Geometry: final body of the model. Coordinates: model frame, mm. A direction names the side the tool comes from. Give positions to 0.01 mm unless a question says otherwise; leave off trailing zeros. Order: outer loops, then holes, each group sorted by start corner. A loop starts at its lowest first (then second) coordinate and runs counter-clockwise, first axis right, second up. Notation, with made-up numbers: (-2.5, 0.5) -> (3.5, 0.5) arc R12 ccw to (3.5, 19.5) -> close; hole circle Ø1 at (-11, -12). An arc over 180 degrees is marked (long way). One line per item, written item: value. Start each with the question number.
```python
from build123d import *

# Parameters (mm, degrees)
BOSS_EXTRU_1_DEPTH      = 6
ESQUISSE3_R             = 0.625
ENL_V_MAT_EXTRU_4_DEPTH = 6
ESQUISSE4_R             = 0.625
ENL_V_MAT_EXTRU_5_DEPTH = 6


with BuildPart() as part:
    # Esquisse1 → Boss.-Extru.1 (new body)
    with BuildSketch(Plane.XY):
        with BuildLine():
            Line((-16, 25.2), (-16, -18.5))
            Line((-16, -18.5), (16, -18.5))
            Line((16, -18.5), (16, 25.161446269))
            ThreePointArc((16, 25.161446269), (-0.008048953, 18.500008258), (-16, 25.2))
        make_face()
        with BuildLine():
            ThreePointArc((-9, -14.5), (-11.121320344, -13.621320344), (-12, -11.5))
            Line((-12, -11.5), (-12, 9.5))
            ThreePointArc((-12, 9.5), (-11.121320344, 11.621320344), (-9, 12.5))
            Line((-9, 12.5), (9, 12.5))
            ThreePointArc((9, 12.5), (11.121320344, 11.621320344), (12, 9.5))
            Line((12, 9.5), (12, -11.5))
            ThreePointArc((12, -11.5), (11.121320344, -13.621320344), (9, -14.5))
            Line((9, -14.5), (-9, -14.5))
        make_face(mode=Mode.SUBTRACT)
    extrude(amount=BOSS_EXTRU_1_DEPTH)

    # Esquisse3 → Enlèv. mat.-Extru.4 (cut)
    with BuildSketch(Plane(origin=(16, 0, 0), x_dir=(0, 0, -1), z_dir=(1, 0, 0))):
        with Locations(Location((-3, -0.5, 0), (0, 0, 90))):
            Circle(ESQUISSE3_R)
        with Locations(Location((-3, -12.5, 0), (0, 0, 90))):
            Circle(ESQUISSE3_R)
    extrude(amount=-ENL_V_MAT_EXTRU_4_DEPTH, mode=Mode.SUBTRACT)

    # Esquisse4 → Enlèv. mat.-Extru.5 (cut)
    with BuildSketch(Plane.ZY.offset(16)):
        with Locations((3.284775488, -12.5)):
            Circle(ESQUISSE4_R)
        with Locations((3.284775488, -0.5)):
            Circle(ESQUISSE4_R)
    extrude(amount=-ENL_V_MAT_EXTRU_5_DEPTH, mode=Mode.SUBTRACT)


solid = part.part
```
1. Cut plane A-A, the plane x = 0. Return loops of the section in (y, z), then the cut area to 3 significant figures.
2. Cut plane B-B, the plane y = 3. Return loops of the section in (x, z), then the cut area to 3 significant figures.
3. Draft query along Y for faces 4 (the cylindrical face through (13.789, -12.996, 2.62)), 5 (the flat face through (0, 13, 0)), 6 (the cylindrical face through (0.2, 18.5, 3)), 7 (the flat face through (0, -18.5, 3)). Return one class per face: pulls with the +Y half, pulls with the -Y half, needs draft (parallel to the pull), parting line crosses it, or undercut.
4. Cut plane D-D, the plane y = -12.5. Return loops of the section in (x, z) (3 decimals), then the cut area to 3 significant figures.
5. Cut plane C-C, the plane z = 1.5. Return loops of the section in (x, y).
6. Access query for faces 1 (the cylindrical face through (14.03, -0.64, 2.39)), 2 (the flat face through (-12, -1, 2)), 3 (the cylindrical face through (-13.79, -13.11, 3.15)). Directions: +Z, -Z, +X, -X, +Y, -Y. A direction counts if a zero-diameter tool reaches every point of the face in a straight line with its end or side. Return the directions, or none.
7. Pin query (flat end, axial travel): P1, Ø3, axis at x = 4, z = 3, coming from the +Y side. Return the tip coordinate at first contact, or that it passes through.
8. Material intervals for L1, parallel to Z at x = 15.15, y = -0.5 (3 decimals); L2, parallel to Y at x = 0.5, z = 5; L3, parallel to Z at x = -15.1, y = -12.5, sorted ascending. Write a range as [from, to].
Answers follow:
1. outline: (-18.5, 0) -> (-14.5, 0) -> (-14.5, 6) -> (-18.5, 6) -> close; (12.5, 0) -> (18.5, 0) -> (18.5, 6) -> (12.5, 6) -> close
1. area: 60.0 mm²
2. outline: (-16, 0) -> (-12, 0) -> (-12, 6) -> (-16, 6) -> close; (12, 0) -> (16, 0) -> (16, 6) -> (12, 6) -> close
2. area: 48.0 mm²
3. face 4: undercut
3. face 5: needs draft
3. face 6: pulls with the +Y half
3. face 7: pulls with the -Y half
4. outline: (-16, 0) -> (-11.828, 0) -> (-11.828, 2.66) -> (-16, 2.66) -> close; (-16, 3.91) -> (-11.828, 3.91) -> (-11.828, 6) -> (-16, 6) -> close; (11.828, 0) -> (16, 0) -> (16, 2.375) -> (11.828, 2.375) -> close; (11.828, 3.625) -> (16, 3.625) -> (16, 6) -> (11.828, 6) -> close
4. area: 39.6 mm²
5. outline: (-16, -18.5) -> (16, -18.5) -> (16, 25.16) arc R22.5 cw to (-16, 25.2) -> close; hole (-12, -11.5) arc R3 ccw to (-9, -14.5) -> (9, -14.5) arc R3 ccw to (12, -11.5) -> (12, 9.5) arc R3 ccw to (9, 12.5) -> (-9, 12.5) arc R3 ccw to (-12, 9.5) -> close
6. face 1: +X
6. face 2: +Z, -Z
6. face 3: -X
7. P1: stops at y = 19.18
8. L1: z = [0, 2.375], [3.625, 6]
8. L2: y = [-18.5, -14.5], [12.5, 18.51]
8. L3: z = [0, 2.66], [3.91, 6]
